Model file for the job. Use its own axes, mm. Face numbers are marked on the shaded views. A direction names the side the tool comes from. Round coordinates to 2 decimals unless told otherwise and drop trailing zeros. Write each loop counter-clockwise with the first axis right and the second up, starting at its lowest first coordinate (ties: lowest second). Pieces come first, ordered by that corner, then holes. Notation, with made-up numbers: (-31, 5.5) - (-10, 5.5) arc R37 ccw to (-10, 41.5) - close; hole circle Ø8 at (4, 79.5). An arc over 180 degrees is marked (long way). One line per item, written item: value.
from build123d import *

# Parameters (mm, degrees)
F0_R          = 0.5
F0_W          = 7
F0_H          = 7
F0_R_2        = 5
F0_W_2        = 2.5
F0_H_2        = 8
F1_DEPTH      = 1.5
F2_DEPTH      = 7.5
F3_DEPTH      = 5
F4_DEPTH      = 2.5
F4_DEPTH_BACK = 3
F5_START      = 1.5
F0_W_3        = 6
F5_DEPTH      = 1


with BuildPart() as f1:
    # F0 (on Top) → F1 (new body)
    with BuildSketch(Plane.XY):
        Polygon((16.25, 8.125), (-16.25, 8.125), (-16.25, 4), (-13.75, 4), (-13.75, -4), (-16.25, -4), (-16.25, -8.125), (16.25, -8.125), align=None)
        with Locations((-15.25, -7.125)):
            Circle(F0_R, mode=Mode.SUBTRACT)
        with Locations((15.25, -7.125)):
            Circle(F0_R, mode=Mode.SUBTRACT)
        with Locations((-15.25, 7.125)):
            Circle(F0_R, mode=Mode.SUBTRACT)
        with Locations((0.75, 3.625)):
            Rectangle(F0_W, F0_H, mode=Mode.SUBTRACT)
        with Locations((10.25, 2.125)):
            Circle(F0_R_2, mode=Mode.SUBTRACT)
        with Locations((15.25, 7.125)):
            Circle(F0_R, mode=Mode.SUBTRACT)
        with Locations((-15, 0)):
            Rectangle(F0_W_2, F0_H_2)
        with Locations((0.75, 3.625)):
            Rectangle(F0_W, F0_H)
        with Locations((10.25, 2.125)):
            Circle(F0_R_2)
    extrude(amount=-F1_DEPTH)

    # F0 (on Top) → F2 (join)
    with BuildSketch(Plane.XY):
        with Locations((10.25, 2.125)):
            Circle(F0_R_2)
    extrude(amount=F2_DEPTH)

    # F0 (on Top) → F3 (join)
    with BuildSketch(Plane.XY):
        with Locations((0.75, 3.625)):
            Rectangle(F0_W, F0_H)
    extrude(amount=F3_DEPTH)

    # F0 (on Top) → F4 (join, two sides)
    with BuildSketch(Plane.XY) as f4_sk:
        with Locations((-15, 0)):
            Rectangle(F0_W_2, F0_H_2)
    extrude(amount=F4_DEPTH)
    extrude(f4_sk.sketch, amount=-F4_DEPTH_BACK)

    # F0 (on Top) → F5 (join)
    with BuildSketch(Plane.XY.offset(F5_START)):
        with Locations((-19.25, 0)):
            Rectangle(F0_W_3, F0_H_2)
    extrude(amount=F5_DEPTH)


solid = f1.part
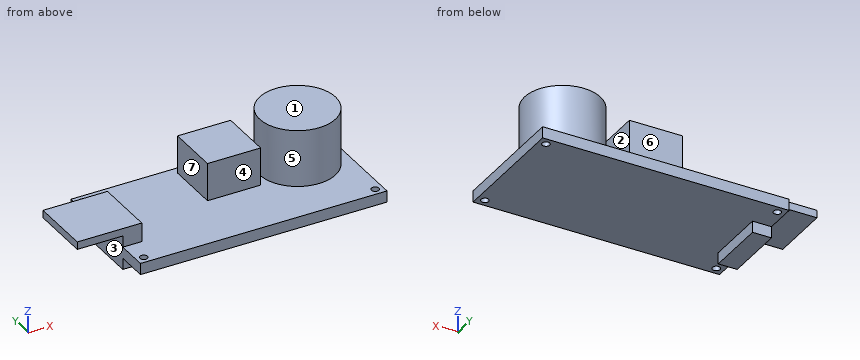
1. Mould opens along X. For the marked faces 1, 2, 3 and 4 say: released by +X, released by -X, zero draft, split by the parting line, or undercut.
Report:
face 1: zero draft
face 2: undercut
face 3: released by -X
face 4: undercut
2. Band-saw the part on A-A on x = -15.25. Write the cut outline in (y, z) (3 decimals).
Report:
outline: (-8.125, -1.5) - (-7.625, -1.5) - (-7.625, 0) - (-8.125, 0) - close; (-6.625, -1.5) - (-4, -1.5) - (-4, -3) - (4, -3) - (4, -1.5) - (6.625, -1.5) - (6.625, 0) - (4, 0) - (4, 2.5) - (-4, 2.5) - (-4, 0) - (-6.625, 0) - close; (7.625, -1.5) - (8.125, -1.5) - (8.125, 0) - (7.625, 0) - close
3. Band-saw the part on D-D on z = 3.5. Write the cut outline in (x, y) (3 decimals).
Report:
outline: (-2.75, 0.125) - (4.25, 0.125) - (4.25, 7.125) - (-2.75, 7.125) - close; circle Ø10 at (10.25, 2.125)
4. Band-saw the part on C-C on y = 5.75. Write the cut outline in (x, z).
Report:
outline: (-16.25, -1.5) - (16.25, -1.5) - (16.25, 0) - (13.69, 0) - (13.69, 7.5) - (6.81, 7.5) - (6.81, 0) - (4.25, 0) - (4.25, 5) - (-2.75, 5) - (-2.75, 0) - (-16.25, 0) - close
5. Tool access for the marked faces 5, 6 and 7: list every direction of +Z, -Z, +X, -X, +Y, -Y with a clear straight run to the whole face (end or side of a thin tool).
Report:
face 5: +Z
face 6: +Z, +X, -X, +Y
face 7: +Z, +Y, -Y
6. Wall check: probe 1 along Y at (x, z) = (15.25, -0.4) (3 decimals); probe 2 along X at (y, z) = (2, 4); probe 3 along Z at (x, y) = (13, -5.5). Give the ranges that are in metal, low to high. Write a range as [from, to].
Report:
probe 1: [-8.125, -7.625], [-6.625, 6.625], [7.625, 8.125]
probe 2: [-2.75, 4.25], [5.25, 15.25]
probe 3: [-1.5, 0]
7. Drop flat-ended pins along their axis: pin 1 (7.5 mm diameter, centred on x = -0.5, y = 4.5, fed in from +Z); pin 2 (5 mm diameter, centred on x = -5, y = 2, fed in from -Z); pin 3 (1.2 mm diameter, centred on y = 1.5, z = 1, fed in from +X). Give the stop position or say it passes through.
Report:
pin 1: z = 5
pin 2: z = -1.5
pin 3: x = 15.25
8. Band-saw the part on B-B on x = 10.25. Write the cut outline in (y, z) (3 decimals), plus the area to 3 significant figures.
Report:
outline: (-8.125, -1.5) - (8.125, -1.5) - (8.125, 0) - (7.125, 0) - (7.125, 7.5) - (-2.875, 7.5) - (-2.875, 0) - (-8.125, 0) - close
area: 99.4 mm²
